Part print with two shaded views. Sizes in mm from the minimum x, y, z corner. A direction names the side the tool comes from. Round coordinates to 2 decimals unless told otherwise and drop trailing zeros. Loops run counter-clockwise (first coordinate to the right, second up) from the corner with the lowest first, then second, coordinate; pieces in that order, holes last. Notation, with made-up numbers: (-20.5, 18) -> (-15.5, 18) arc R21 cw to (-15.5, 45) -> close; hole circle Ø7 at (36, -37). An arc over 180 degrees is marked (long way). Put each result on its own line as item: value. Start each with the question number.
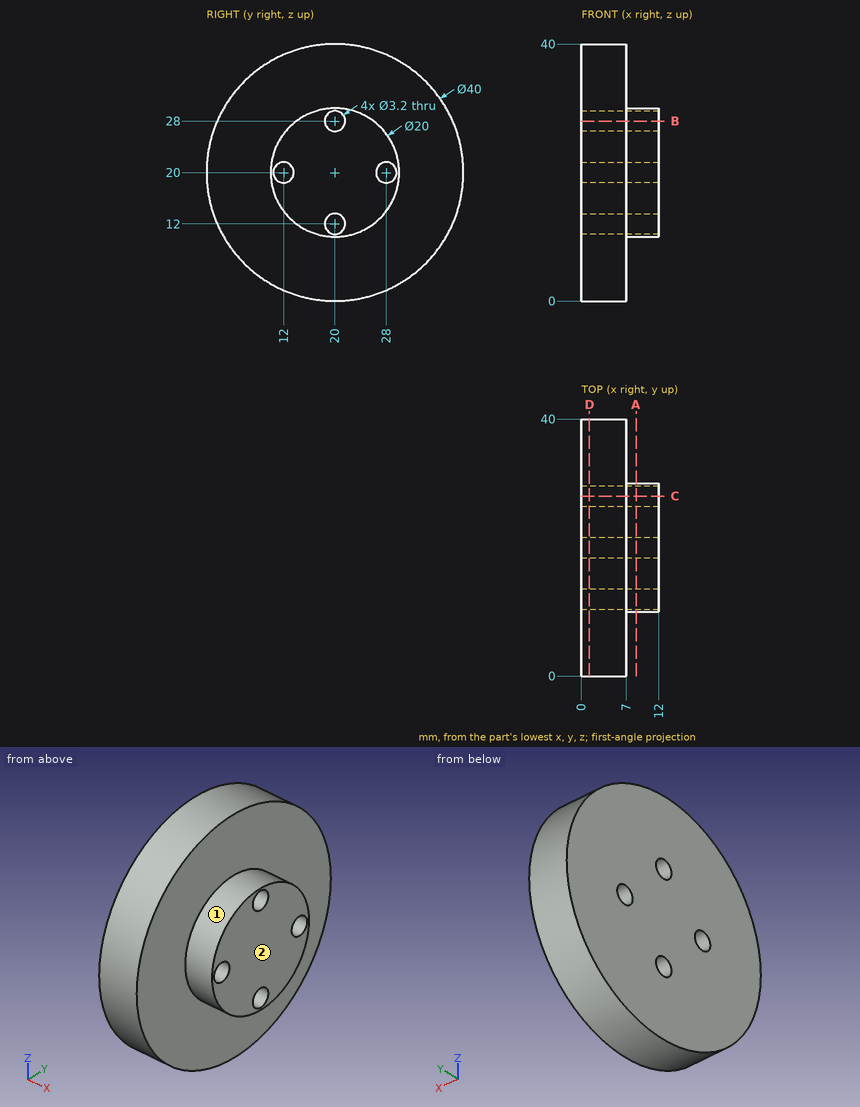
Item 1: Cut at B-B on z = 28. Write the cut outline in (x, y).
Item 2: 3-axis set-ups, long thin cutter, end or side, ignore diameter. For the marked faces 1 and 2: which of +Z, -Z, +X, -X, +Y, -Y reach the whole face in a straight line?
Item 3: Cut at D-D on x = 1.25. Write the cut outline in (y, z).
Item 4: Drop flat-ended pins along their axis: pin 1 (3 mm diameter, centred on y = 5.5, z = 7.5, fed in from +X); pin 2 (1.5 mm diameter, centred on x = 7.5, y = 20, fed in from -Z); pin 3 (4 mm diameter, centred on x = 3.5, z = 22.5, fed in from +Y). Give the stop position or say it passes through.
Item 5: Cut at A-A on x = 8.5. Write the cut outline in (y, z).
Item 6: Wall check: line 1 (X direction, y = 24.5, z = 10); line 2 (Y direction, x = 3.25, z = 11); line 3 (Y direction, x = 6.25, z = 32). Give the ranges that are in metal, low to high. Write a range as from..to.
Ans:
1. outline: (0, 1.67) -> (7, 1.67) -> (7, 14) -> (12, 14) -> (12, 18.4) -> (0, 18.4) -> close; (0, 21.6) -> (12, 21.6) -> (12, 26) -> (7, 26) -> (7, 38.33) -> (0, 38.33) -> close
2. face 1: +X
2. face 2: +Z, -Z, +X, +Y, -Y
3. outline: circle Ø40 at (20, 20); hole circle Ø3.2 at (12, 20); hole circle Ø3.2 at (20, 12); hole circle Ø3.2 at (20, 28); hole circle Ø3.2 at (28, 20)
4. pin 1: stops at x = 7
4. pin 2: stops at z = 0
4. pin 3: stops at y = 39.99
5. outline: circle Ø20 at (20, 20); hole circle Ø3.2 at (12, 20); hole circle Ø3.2 at (20, 12); hole circle Ø3.2 at (20, 28); hole circle Ø3.2 at (28, 20)
6. line 1: x = 0..7
6. line 2: y = 2.14..18.75, 21.25..37.86
6. line 3: y = 4..36
